Geometry: final body of the model. Coordinates: model frame, mm. A direction names the side the tool comes from. Coordinates: 2 decimals unless noted, no trailing zeros. Order: outer loops, then holes, each group sorted by start corner. A loop starts at its lowest first (then second) coordinate and runs counter-clockwise, first axis right, second up. Notation, with made-up numbers: M -40,8.5 L -24,8.5 A25 cw -24,41.5 Z; hole C -34.75,88.5 d3. An arc over 180 degrees is marked long. One line per question, with ' | ' between items.
Autodesk Inventor part; units mm, degrees
ref_plane "位置合わせ" through (-6, 0, -16.25) normal (0, 0, 1) x (1, 0, 0)
ref_plane "YZ Plane" through (0, 0, 0) normal (1, 0, 0) x (0, 1, 0)
ref_plane "XZ Plane" through (0, 0, 0) normal (0, 1, 0) x (-1, 0, 0)
sketch "スケッチ1" plane through (0, 0, 0) normal (0, 1, 0) x (-1, 0, 0)
  line L0 (6, 12.25) -> (-6, 12.25)
  line L1 (-6, 12.25) -> (-6, -12.25)
  line L2 (-6, -12.25) -> (6, -12.25)
  line L3 (6, -12.25) -> (6, 12.25)
  line L4 (9, 19.25) -> (-9, 19.25)
  line L5 (-9, 19.25) -> (-9, -16.25)
  line L6 (-9, -16.25) -> (9, -16.25)
  line L7 (9, -16.25) -> (9, 19.25)
  line L8 (0, -13.75) -> (0, 13.75) construction
  point P0 (0, 0)
  point P1 (6, 0)
  point P2 (0, 12.25)
  point P3 (0, 19.25)
  point P4 (9, 1.5)
  point P5 (0, 0)
  dimension "d0" = 24.5
  dimension "d1" = 12
  dimension "d2" = 3
  dimension "d3" = 4
  dimension "d4" = 7
  dimension "d8" = 27.5
extrude "押し出し1" add sketch "スケッチ1" along normal blind 2
hole "穴1" at (0, 0, -13.75) at (0, 0, 13.75) direction (0, 1, 0) diameter 1.5 end through all
mirror "ミラー1" about plane through (9, 0, -16.25) normal (0, 0, -1) of "押し出し1", "穴1"
fillet "フィレット1" radius 5 4 edges at (-9, 1, 19.25) (9, 1, 19.25) (9, 1, -51.75) (-9, 1, -51.75)
ref_plane "位置合わせ" through (-6, 0, -16.25) normal (0, 0, 1) x (1, 0, 0)
sketch "スケッチ2" plane through (0, 2, 0) normal (0, 1, 0) x (1, 0, 0)
  line L0 (-9, -14.25) -> (-9, 46.75)
  line L1 (9, -14.25) -> (9, 46.75)
  circle A0 centre (0, 18.75) radius 0.75
  circle A1 centre (0, 13.75) radius 0.75
  circle A2 centre (7.5, 16.25) radius 1.5
  circle A3 centre (-7.5, 16.25) radius 1.5
  line L2 (0, 18.75) -> (0, 13.75) construction
  point P0 (0, 0)
  point P1 (0, 16.25)
  dimension "d16" = 3
extrude "押し出し2" add sketch "スケッチ2" along normal blind 1 contours A2 | A3
properties part number "ServoMotor_Holder_V2"
1. Access query for faces 1 (the face through (0, 1, -12.25)), 2 (the face through (0, 2, -17)), 3 (the face through (-9, 1, -17)). Directions: +Z, -Z, +X, -X, +Y, -Y. A direction counts if a zero-diameter tool reaches every point of the face in a straight line with its end or side. Return the directions, or none.
Response values:
face 1: +Y, -Y | face 2: +Y | face 3: +Z, -Z, -X, +Y, -Y
2. Material intervals for line 1 (Z direction, x = 1.25, y = 1.9); line 2 (X direction, y = 1.65, z = 4.5); line 3 (X direction, y = 0.65, z = -18.75), sorted ascending. Write a range as [from, to].
Response values:
line 1: z = [-51.75, -44.75], [-20.25, -12.25], [12.25, 19.25] | line 2: x = [-9, -6], [6, 9] | line 3: x = [-9, -0.75], [0.75, 9]
3. Section A-A, the plane z = -11. Output: boundary loops of the cut face in (x, y).
Response values:
outline: M -9,0 L -6,0 L -6,2 L -9,2 Z; M 6,0 L 9,0 L 9,2 L 6,2 Z
4. Section C-C, the plane y = 1.5. Output: boundary loops of the cut face in (x, z).
Response values:
outline: M -9,-46.75 A5 ccw -4,-51.75 L 4,-51.75 A5 ccw 9,-46.75 L 9,14.25 A5 ccw 4,19.25 L -4,19.25 A5 ccw -9,14.25 Z; hole M -6,-44.75 L 6,-44.75 L 6,-20.25 L -6,-20.25 Z; hole M -6,-12.25 L 6,-12.25 L 6,12.25 L -6,12.25 Z; hole C 0,-46.25 d1.5; hole C 0,-18.75 d1.5; hole C 0,-13.75 d1.5; hole C 0,13.75 d1.5
5. Draft query along X for faces 4 (the face through (-8, 3, -16)), 5 (the face through (-7.5, 1.01, -50.32)), 6 (the face through (-0.456, 1.014, -19.345)). Return one class per face: pulls with the +X half, pulls with the -X half, needs draft (parallel to the pull), parting line crosses it, or undercut.
Response values:
face 4: needs draft | face 5: pulls with the -X half | face 6: undercut
6. Pin query (flat end, axial travel): P1, Ø1.4, axis at x = 0, z = -13.75, coming from the -Y side; P2, Ø1.5, axis at x = 6.5, y = 2.5, coming from the +Z side; P3, Ø1.5, axis at x = 2.5, z = -12, coming from the +Y side. Return the tip coordinate at first contact, or that it passes through.
Response values:
P1: passes through | P2: stops at z = 18.86 | P3: stops at y = 2
7. Section B-B, the plane x = 5. Output: boundary loops of the cut face in (y, z).
Response values:
outline: M 0,-51.65 L 2,-51.65 L 2,-44.75 L 0,-44.75 Z; M 0,-20.25 L 2,-20.25 L 2,-12.25 L 0,-12.25 Z; M 0,12.25 L 2,12.25 L 2,19.15 L 0,19.15 Z
